Work out the finished part from the listing and answer in its coordinate system (mm). Coordinates: 2 decimals unless noted, no trailing zeros. Write each loop counter-clockwise with the first axis right and the second up, starting at its lowest first coordinate (ties: lowest second). Pieces come first, ordered by that corner, then holes. Notation, with made-up numbers: (-4, 87.5) - (50, 87.5) arc R4 cw to (50, 92.5) - close; hole circle Ø8 at (43, 1). An arc over 180 degrees is marked (long way). One line per item, written item: value.
```python
from build123d import *

# Parameters (mm, degrees)
BOSS_EXTRUDE1_DEPTH = 6.35
FILLET1_R           = 2
SKETCH2_R           = 1.5
SKETCH2_W           = 6.35
SKETCH2_H           = 50
SKETCH2_W_2         = 120
SKETCH2_H_2         = 120
CUT_EXTRUDE1_DEPTH  = 6.35
FILLET2_R           = 10


with BuildPart() as part:
    # Sketch1 → Boss-Extrude1 (new body)
    with BuildSketch(Plane(origin=(0, 0, 0), x_dir=(1, 0, 0), z_dir=(0, 1, 0))):
        Polygon((0, 0), (295, 0), (295, 59), (301.35, 59), (301.35, 109), (295, 109), (295, 169), (301.35, 169), (301.35, 219), (295, 219), (295, 279), (301.35, 279), (301.35, 329), (295, 329), (295, 389), (301.35, 389), (301.35, 439), (295, 439), (295, 499), (301.35, 499), (301.35, 549), (295, 549), (295, 609), (0, 609), (0, 549), (-6.35, 549), (-6.35, 499), (0, 499), (0, 439), (-6.35, 439), (-6.35, 389), (0, 389), (0, 329), (-6.35, 329), (-6.35, 279), (0, 279), (0, 219), (-6.35, 219), (-6.35, 169), (0, 169), (0, 109), (-6.35, 109), (-6.35, 59), (0, 59), align=None)
    extrude(amount=BOSS_EXTRUDE1_DEPTH)

    # Fillet1
    fillet1_edges = [part.edges().sort_by_distance(p)[0] for p in [
        (-6.35, 3.175, -59),
        (-6.35, 3.175, -109),
        (-6.35, 3.175, -169),
        (-6.35, 3.175, -219),
        (-6.35, 3.175, -279),
        (-6.35, 3.175, -329),
        (-6.35, 3.175, -389),
        (-6.35, 3.175, -439),
        (-6.35, 3.175, -499),
        (-6.35, 3.175, -549),
        (301.35, 3.175, -549),
        (301.35, 3.175, -499),
        (301.35, 3.175, -439),
        (301.35, 3.175, -389),
        (301.35, 3.175, -329),
        (301.35, 3.175, -279),
        (301.35, 3.175, -219),
        (301.35, 3.175, -169),
        (301.35, 3.175, -109),
        (301.35, 3.175, -59),
    ]]
    fillet(fillet1_edges, radius=FILLET1_R)

    # Sketch2 → Cut-Extrude1 (cut)
    with BuildSketch(Plane(origin=(0, 6.35, 0), x_dir=(1, 0, 0), z_dir=(0, 1, 0))):
        with Locations(Location((15, 15, 0), (0, 0, 270))):
            Circle(SKETCH2_R)
        with Locations(Location((251.65, 15, 0), (0, 0, 270))):
            Circle(SKETCH2_R)
        with Locations(Location((15, 131.925897501, 0), (0, 0, 270))):
            Circle(SKETCH2_R)
        with Locations((269.825, 194)):
            Rectangle(SKETCH2_W, SKETCH2_H)
        with Locations((269.825, 84)):
            Rectangle(SKETCH2_W, SKETCH2_H)
        with BuildLine():
            Line((55.042435698, 504.435466218), (111.042435698, 504.435466218))
            ThreePointArc((111.042435698, 504.435466218), (115.992183166, 502.385213686), (118.042435698, 497.435466218))
            Line((118.042435698, 497.435466218), (118.042435698, 441.435466218))
            ThreePointArc((118.042435698, 441.435466218), (115.992183166, 436.48571875), (111.042435698, 434.435466218))
            Line((111.042435698, 434.435466218), (55.042435698, 434.435466218))
            ThreePointArc((55.042435698, 434.435466218), (50.09268823, 436.48571875), (48.042435698, 441.435466218))
            Line((48.042435698, 441.435466218), (48.042435698, 497.435466218))
            ThreePointArc((48.042435698, 497.435466218), (50.09268823, 502.385213686), (55.042435698, 504.435466218))
        make_face()
        with BuildLine():
            Line((185.233522799, 503.969461472), (241.233522799, 503.969461472))
            ThreePointArc((241.233522799, 503.969461472), (246.183270267, 501.91920894), (248.233522799, 496.969461472))
            Line((248.233522799, 496.969461472), (248.233522799, 440.969461472))
            ThreePointArc((248.233522799, 440.969461472), (246.183270267, 436.019714004), (241.233522799, 433.969461472))
            Line((241.233522799, 433.969461472), (185.233522799, 433.969461472))
            ThreePointArc((185.233522799, 433.969461472), (180.283775331, 436.019714004), (178.233522799, 440.969461472))
            Line((178.233522799, 440.969461472), (178.233522799, 496.969461472))
            ThreePointArc((178.233522799, 496.969461472), (180.283775331, 501.91920894), (185.233522799, 503.969461472))
        make_face()
        with BuildLine():
            Line((43.325, 239.143159068), (83.325, 239.143159068))
            ThreePointArc((83.325, 239.143159068), (90.396067812, 236.21422688), (93.325, 229.143159068))
            Line((93.325, 229.143159068), (93.325, 189.143159068))
            ThreePointArc((93.325, 189.143159068), (90.396067812, 182.072091256), (83.325, 179.143159068))
            Line((83.325, 179.143159068), (43.325, 179.143159068))
            ThreePointArc((43.325, 179.143159068), (36.253932188, 182.072091256), (33.325, 189.143159068))
            Line((33.325, 189.143159068), (33.325, 229.143159068))
            ThreePointArc((33.325, 229.143159068), (36.253932188, 236.21422688), (43.325, 239.143159068))
        make_face()
        with Locations((67.172717051, 313.959589149)):
            Rectangle(SKETCH2_W_2, SKETCH2_H_2)
        with Locations((219.464803824, 313.959589149)):
            Rectangle(SKETCH2_W_2, SKETCH2_H_2)
        with BuildLine():
            Line((173.325, 229.143159068), (173.325, 189.143159068))
            ThreePointArc((173.325, 189.143159068), (176.253932188, 182.072091256), (183.325, 179.143159068))
            Line((183.325, 179.143159068), (223.325, 179.143159068))
            ThreePointArc((223.325, 179.143159068), (230.396067812, 182.072091256), (233.325, 189.143159068))
            Line((233.325, 189.143159068), (233.325, 229.143159068))
            ThreePointArc((233.325, 229.143159068), (230.396067812, 236.21422688), (223.325, 239.143159068))
            Line((223.325, 239.143159068), (183.325, 239.143159068))
            ThreePointArc((183.325, 239.143159068), (176.253932188, 236.21422688), (173.325, 229.143159068))
        make_face()
    extrude(amount=-CUT_EXTRUDE1_DEPTH, mode=Mode.SUBTRACT)

    # Fillet2
    fillet2_edges = [part.edges().sort_by_distance(p)[0] for p in [
        (7.172717051, 3.175, -253.959589149),
        (7.172717051, 3.175, -373.959589149),
        (127.172717051, 3.175, -373.959589149),
        (127.172717051, 3.175, -253.959589149),
        (159.464803824, 3.175, -253.959589149),
        (159.464803824, 3.175, -373.959589149),
        (279.464803824, 3.175, -373.959589149),
        (279.464803824, 3.175, -253.959589149),
    ]]
    fillet(fillet2_edges, radius=FILLET2_R)


solid = part.part
```
Item 1: Consider probe 1 along X at (y, z) = (2.75, -15); probe 2 along X at (y, z) = (4.75, -363); probe 3 along Z at (x, y) = (107, 0.75). Determine where each line is inside the solid, lowest interval first.
Evaluation:
probe 1: x = 0 to 13.5, 16.5 to 250.15, 253.15 to 295
probe 2: x = 0 to 7.17, 127.17 to 159.46, 279.46 to 295
probe 3: z = -609 to -504.44, -434.44 to -373.96, -253.96 to 0
Item 2: Section B-B, the plane z = -74.5 is taken. Determine the outline of the cut face in (x, y), then the cut area to 3 significant figures.
Evaluation:
outline: (-6.35, 0) - (266.65, 0) - (266.65, 6.35) - (-6.35, 6.35) - close; (273, 0) - (301.35, 0) - (301.35, 6.35) - (273, 6.35) - close
area: 1,910 mm2
Item 3: Given pin 1 (1.5 mm diameter, centred on y = 4.5, z = -382, fed in from -X); pin 2 (1.3 mm diameter, centred on x = 296.5, y = 2.5, fed in from +Z); pin 3 (1.9 mm diameter, centred on y = 2.5, z = -16.5, fed in from +X), each flat-ended and moving along its own axis, determine where each tip first touches the part or whether it passes through.
Evaluation:
pin 1: stops at x = 0
pin 2: stops at z = -59
pin 3: stops at x = 295
Item 4: Section A-A, the plane z = -470.5 is taken. Determine the outline of the cut face in (x, y).
Evaluation:
outline: (0, 0) - (48.04, 0) - (48.04, 6.35) - (0, 6.35) - close; (118.04, 0) - (178.23, 0) - (178.23, 6.35) - (118.04, 6.35) - close; (248.23, 0) - (295, 0) - (295, 6.35) - (248.23, 6.35) - close
Item 5: Section C-C, the plane y = 3.75 is taken. Give the number of separate pieces and of enclosed holes in the cut face, then the cut area to 3 significant figures.
Evaluation:
separate pieces: 1
enclosed holes: 11
area: 137,000 mm2
